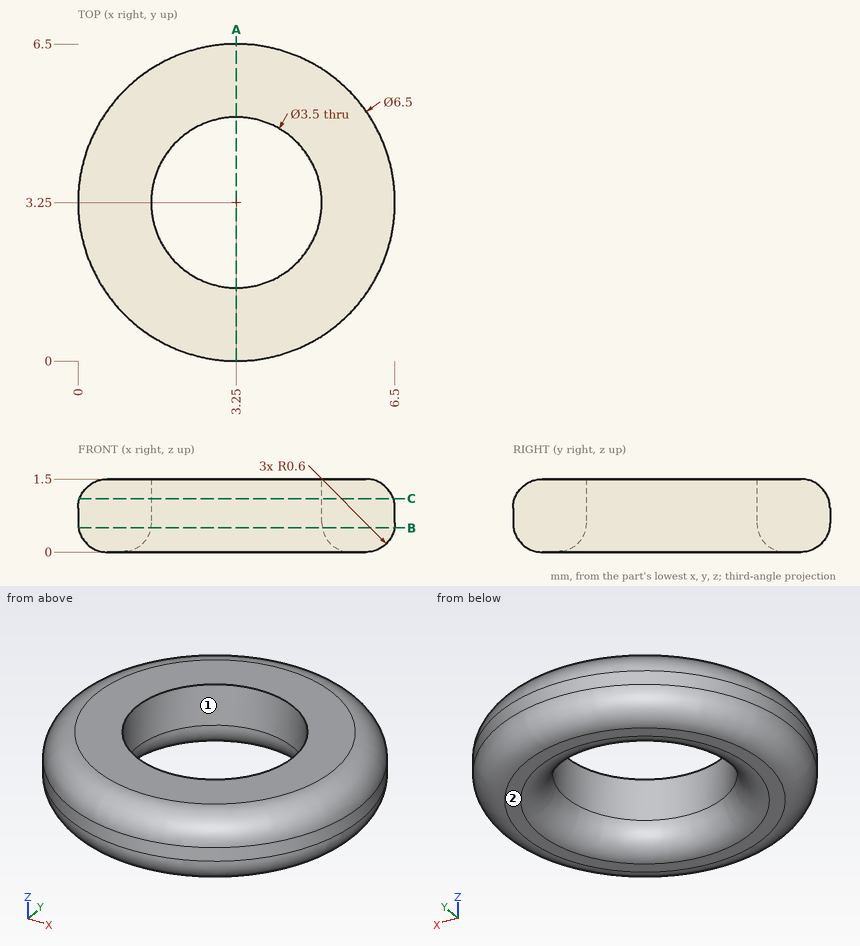
Geometry: see drawing. Coordinates: mm, zero at the bounding-box minimum. Give positions to 0.01 mm unless a question says otherwise; leave off trailing zeros. Order: outer loops, then holes, each group sorted by start corner. A loop starts at its lowest first (then second) coordinate and runs counter-clockwise, first axis right, second up.
1. Cut plane A-A (x = 3.25). Return loops of the section in (y, z).
Computed:
outline: (0, 0.6) arc R0.6 ccw to (0.6, 0) - (0.9, 0) arc R0.6 ccw to (1.5, 0.6) - (1.5, 1.5) - (0.6, 1.5) arc R0.6 ccw to (0, 0.9) - close; (5, 0.6) arc R0.6 ccw to (5.6, 0) - (5.9, 0) arc R0.6 ccw to (6.5, 0.6) - (6.5, 0.9) arc R0.6 ccw to (5.9, 1.5) - (5, 1.5) - close
2. Line query: probe 1 along Y at (x, z) = (3.5, 1.1); probe 2 along X at (y, z) = (3.5, 0.15); probe 3 along X at (y, z) = (3.75, 1.35). Output: solid intervals per line, ascending.
Computed:
probe 1: y = 0.04 to 1.52, 4.98 to 6.46
probe 2: x = 0.21 to 1.31, 5.19 to 6.29
probe 3: x = 0.24 to 1.57, 4.93 to 6.26
3. Cut plane B-B (z = 0.5). Return loops of the section in (x, y).
Computed:
outline: circle Ø6.48 at (3.25, 3.25); hole circle Ø3.52 at (3.25, 3.25)
4. Cut plane C-C (z = 1.1). Return loops of the section in (x, y).
Computed:
outline: circle Ø6.43 at (3.25, 3.25); hole circle Ø3.5 at (3.25, 3.25)
5. Draft query along Y for the marked faces 1 and 2. Return one class per face: released by +Y, released by -Y, zero draft, split by the parting line, or undercut.
Computed:
face 1: undercut
face 2: zero draft
